from build123d import *

# Parameters (mm, degrees)
SKETCH1_R               = 8.5
BOSS_EXTRUDE1_DEPTH     = 16.2
SKETCH4_W               = 0.7
SKETCH4_H               = 17
CUT_EXTRUDE2_DEPTH      = 21.172753902
SKETCH5_R               = 15
BOSS_EXTRUDE2_DEPTH     = 4
BOSS_EXTRUDE3_DEPTH     = 16
SKETCH7_R               = 1.85
CUT_EXTRUDE3_DEPTH      = 30.292319813
CHAMFER1_SIZE           = 0.5
CUT_EXTRUDE4_DEPTH      = 42.957597643
CUT_EXTRUDE4_DEPTH_BACK = 42.957597643
SKETCH8_R               = 1.25
CUT_EXTRUDE5_DEPTH      = 44.121224472
SKETCH10_R              = 2.1
CUT_EXTRUDE6_DEPTH      = 44.121224472
FILLET1_R               = 0.5
CHAMFER2_SIZE           = 1


with BuildPart() as part:
    # Sketch1 → Boss-Extrude1 (new body)
    with BuildSketch(Plane(origin=(0, 0, 0), x_dir=(0, 0, -1), z_dir=(1, 0, 0))):
        Circle(SKETCH1_R)
        with BuildLine():
            Line((2.4, 1.882153022), (2.4, -1.882153022))
            ThreePointArc((2.4, -1.882153022), (-3.05, 0), (2.4, 1.882153022))
        make_face(mode=Mode.SUBTRACT)
    extrude(amount=BOSS_EXTRUDE1_DEPTH)

    # Sketch4 → Cut-Extrude2 (cut, through all)
    with BuildSketch(Plane.ZY):
        Rectangle(SKETCH4_W, SKETCH4_H)
    extrude(amount=-CUT_EXTRUDE2_DEPTH, mode=Mode.SUBTRACT)


with BuildPart() as cut_extrude2_piece_1:
    # of the separate pieces the step leaves, piece 1, a body of its own (cut_extrude2_pieces)
    add(part.part.solids().sort_by_distance((0, -8.492791061, -0.35))[0])



with BuildPart() as cut_extrude2_piece_2:
    # of the separate pieces the step leaves, piece 2, a body of its own (cut_extrude2_pieces)
    add(part.part.solids().sort_by_distance((0, 3.029851482, 0.35))[0])


with BuildPart() as cut_extrude2_piece_1_1:
    add(cut_extrude2_piece_1.part)

    add(cut_extrude2_piece_2.part)  # Boss-Extrude2 merges Cut-Extrude2 piece 2
    # Sketch5 → Boss-Extrude2 (add)
    with BuildSketch(Plane(origin=(16.2, 0, 0), x_dir=(0, 0, -1), z_dir=(1, 0, 0))):
        Circle(SKETCH5_R)
    extrude(amount=BOSS_EXTRUDE2_DEPTH)

    # Sketch6 → Boss-Extrude3 (add)
    with BuildSketch(Plane(origin=(20.2, 0, 0), x_dir=(0, 0, -1), z_dir=(1, 0, 0))):
        Polygon((2.343936023, 5.658762137), (-2.343936023, 5.658762137), (-5.658762137, 2.343936023), (-5.658762137, -2.343936023), (-2.343936023, -5.658762137), (2.343936023, -5.658762137), (5.658762137, -2.343936023), (5.658762137, 2.343936023), align=None)
    extrude(amount=BOSS_EXTRUDE3_DEPTH)

    # Sketch7 → Cut-Extrude3 (cut, through all)
    with BuildSketch(Plane(origin=(20.2, 0, 0), x_dir=(0, 0, -1), z_dir=(1, 0, 0))):
        with Locations((0, 11.5)):
            Circle(SKETCH7_R)
        with Locations((-9.959292144, -5.75)):
            Circle(SKETCH7_R)
        with Locations((9.959292144, -5.75)):
            Circle(SKETCH7_R)
    extrude(amount=-CUT_EXTRUDE3_DEPTH, mode=Mode.SUBTRACT)

    # Chamfer1
    chamfer1_edges = [cut_extrude2_piece_1_1.edges().sort_by_distance(p)[0] for p in [
        (36.2, 4.00134908, -4.00134908),
        (36.2, 5.658762137, 0),
        (36.2, 4.00134908, 4.00134908),
        (36.2, 0, 5.658762137),
        (36.2, -4.00134908, 4.00134908),
        (36.2, -5.658762137, 0),
        (36.2, -4.00134908, -4.00134908),
        (36.2, 0, -5.658762137),
    ]]
    chamfer(chamfer1_edges, length=CHAMFER1_SIZE)

    # Sketch8 → Cut-Extrude4 (cut, two sides: drawn at the far end of the back side and taken through both)
    with BuildSketch(Plane.XY.offset(-CUT_EXTRUDE4_DEPTH_BACK)):
        with Locations((6, 6)):
            Circle(SKETCH8_R)
        with Locations((6, -6)):
            Circle(SKETCH8_R)
    extrude(amount=CUT_EXTRUDE4_DEPTH + CUT_EXTRUDE4_DEPTH_BACK, mode=Mode.SUBTRACT)

    # Sketch9 → Cut-Extrude5 (cut, through all)
    with BuildSketch(Plane.XY.offset(3)):
        Polygon((7.241303079, 3.85), (8.482606158, 6), (7.241303079, 8.15), (4.758696921, 8.15), (3.517393842, 6), (4.758696921, 3.85), align=None)
        Polygon((7.241303079, -8.15), (8.482606158, -6), (7.241303079, -3.85), (4.758696921, -3.85), (3.517393842, -6), (4.758696921, -8.15), align=None)
    extrude(amount=CUT_EXTRUDE5_DEPTH, mode=Mode.SUBTRACT)

    # Sketch10 → Cut-Extrude6 (cut, through all)
    with BuildSketch(Plane.XY.offset(-3)):
        with Locations((6, 6)):
            Circle(SKETCH10_R)
        with Locations((6, -6)):
            Circle(SKETCH10_R)
    extrude(amount=-CUT_EXTRUDE6_DEPTH, mode=Mode.SUBTRACT)

    # Fillet1
    fillet1_edges = [cut_extrude2_piece_1_1.edges().sort_by_distance(p)[0] for p in [
        (16.2, 0, 8.5),
        (16.2, 0, -8.5),
    ]]
    fillet(fillet1_edges, radius=FILLET1_R)

    # Chamfer2
    chamfer2_edges = [cut_extrude2_piece_1_1.edges().sort_by_distance(p)[0] for p in [
        (20.2, 4.00134908, -4.00134908),
        (20.2, 5.658762137, 0),
        (20.2, 4.00134908, 4.00134908),
        (20.2, 0, 5.658762137),
        (20.2, -4.00134908, 4.00134908),
        (20.2, -5.658762137, 0),
        (20.2, -4.00134908, -4.00134908),
        (20.2, 0, -5.658762137),
    ]]
    chamfer(chamfer2_edges, length=CHAMFER2_SIZE)


solid = cut_extrude2_piece_1_1.part
Model file for the job. Use its own axes, mm. A direction names the side the tool comes from. Coordinates: 2 decimals unless noted, no trailing zeros. Loops run counter-clockwise (first coordinate to the right, second up) from the corner with the lowest first, then second, coordinate; pieces in that order, holes last. Notation, with made-up numbers: (28, -21.5) -> (41, -21.5) arc R16 cw to (41, -1.5) -> close; hole circle Ø8 at (-35.75, 2.5). An arc over 180 degrees is marked (long way). Use one line per item in the form item = value. Start each with the question number.
(1) Flat gauge pins, fed straight in: pin 1 (5 mm diameter, centred on y = 11.5, z = 0, fed in from -X); pin 2 (6 mm diameter, centred on x = 6.5, y = 3.5, fed in from +Z); pin 3 (6 mm diameter, centred on y = 9.5, z = 2, fed in from +X); pin 4 (2 mm diameter, centred on y = -5.75, z = -9.96, fed in from -X). Where does each tip first touch, or does it go through?
(2) Cut at B-B on y = 0. Give the cut face in (x, z), and give its area (3 significant figures).
(3) Cut at C-C on x = 31.5. Give the cut face in (y, z), and give its area (3 significant figures).
(4) Pull direction Z, two halves, no side cores. Call faces 5 (the flat face through (8, -5, -0.35)), 6 (the flat face through (5, -7, -3)), 7 (the flat face through (7.87, -4.94, 4.75)): pulls with the +Z half, pulls with the -Z half, needs draft (parallel to the pull), parting line crosses it, or undercut.
(5) Probe probe 1 along Y at (x, z) = (6, 1.25); probe 2 along Y at (x, z) = (6, 2.4); probe 3 along X at (y, z) = (6, -5.75). List the from-to ranges inside material, lowest first. Write a range as from..to.
(6) Tool access for faces 1 (the flat face through (16.2, 0, 0)), 2 (the flat face through (7.853, 4.91, 4.748)), 3 (the flat face through (28, 5.659, 0)), 4 (the flat face through (8, 5, 0.35)): list every direction of +Z, -Z, +X, -X, +Y, -Y with a clear straight run to the whole face (end or side of a thin tool).
(7) Cut at D-D on y = 11.5. Give the cut face in (x, z), and give its area (3 significant figures).
Values:
q1.pin_1 = 16.2
q1.pin_2 = 8.49
q1.pin_3 = 20.36
q1.pin_4 = through
q2.outline = (0, -8.5) -> (15.7, -8.5) arc R0.5 cw to (16.2, -9) -> (16.2, -15) -> (20.2, -15) -> (20.2, -6.66) -> (21.2, -5.66) -> (35.7, -5.66) -> (36.2, -5.16) -> (36.2, 5.16) -> (35.7, 5.66) -> (21.2, 5.66) -> (20.2, 6.66) -> (20.2, 15) -> (16.2, 15) -> (16.2, 9) arc R0.5 cw to (15.7, 8.5) -> (0, 8.5) -> (0, 3.05) -> (16.2, 3.05) -> (16.2, -2.4) -> (0, -2.4) -> close
q2.area = 489 mm2
q3.outline = (-5.66, -2.34) -> (-2.34, -5.66) -> (2.34, -5.66) -> (5.66, -2.34) -> (5.66, 2.34) -> (2.34, 5.66) -> (-2.34, 5.66) -> (-5.66, 2.34) -> close
q3.area = 106 mm2
q4.face_5 = undercut
q4.face_6 = pulls with the -Z half
q4.face_7 = needs draft
q5.probe_1 = -8.41..-7.25, -4.75..-2.78, 2.78..4.75, 7.25..8.41
q5.probe_2 = -8.15..-7.25, -4.75..-1.88, 1.88..4.75, 7.25..8.15
q5.probe_3 = 0..3.9, 8.1..20.2
q6.face_1 = -X
q6.face_2 = +Z
q6.face_3 = +Z, -Z, +X, +Y
q6.face_4 = -X, +Y, -Y
q7.outline = (16.2, -9.63) -> (20.2, -9.63) -> (20.2, -1.85) -> (16.2, -1.85) -> close; (16.2, 1.85) -> (20.2, 1.85) -> (20.2, 9.63) -> (16.2, 9.63) -> close
q7.area = 62.2 mm2
